Model file for the job. Use its own axes, mm. Coordinates: 2 decimals unless noted, no trailing zeros. Write each loop counter-clockwise with the first axis right and the second up, starting at its lowest first coordinate (ties: lowest second). Pieces come first, ordered by that corner, then holes. Notation, with made-up numbers: (53, 54.25) - (111, 54.25) arc R15 ccw to (111, 69.25) - close; hole circle Ø8 at (-31.5, -8.5). An arc over 180 degrees is marked (long way). Put each result on its own line as item: value. Start each with the question number.
1. Saw through at B-B, the plane y = 137.5. Write the cut outline in (x, z), plus the area to 3 significant figures.
2. Saw through at A-A, the plane z = 9. Write the cut outline in (x, y), plus the area to 3 significant figures.
3. Drop flat-ended pins along their axis: P1, Ø1.5, axis at x = 9.5, y = 92, coming from the +Z side; P2, Ø1, axis at y = 118.5, z = 6, coming from the +X side; P3, Ø4, axis at y = 170.5, z = -11, coming from the -X side. Give the stop position or say it passes through.
4. Saw through at D-D, the plane y = 15. Write the cut outline in (x, z).
5. Saw through at C-C, the plane z = -6.5. Write the cut outline in (x, y).
6. Drill centre lines: L1, parallel to Y at x = 0, z = -4.5; L2, parallel to Y at x = 1, z = 5; L3, parallel to X at y = 15, z = 0. Where is each one in solid material? Low to high. Write a range as from..to.
```python
from build123d import *

# Parameters (mm, degrees)
SKETCH1_W          = 15
SKETCH1_H          = 210
SKETCH3_R          = 3.25
CUT_EXTRUDE1_DEPTH = 212.068709192


with BuildPart() as part:
    # Sketch1 → Revolve1 (revolve)
    with BuildSketch(Plane.XY, mode=Mode.PRIVATE) as revolve1_sk:
        with Locations((-7.5, 105)):
            Rectangle(SKETCH1_W, SKETCH1_H)
    revolve(revolve1_sk.sketch.rotate(Axis((0, 0, 0), (0, 1, 0)), 270), axis=Axis((0, 0, 0), (0, 1, 0)))

    # Sketch3 → Cut-Extrude1 (cut, symmetric)
    with BuildSketch(Plane.XY):
        with Locations((0, 195)):
            Circle(SKETCH3_R)
    cut_extrude1 = extrude(amount=CUT_EXTRUDE1_DEPTH, both=True, mode=Mode.SUBTRACT)

    # Mirror1: Cut-Extrude1 across plane
    add(cut_extrude1.mirror(Plane.ZX.offset(105)), mode=Mode.SUBTRACT)


solid = part.part
```
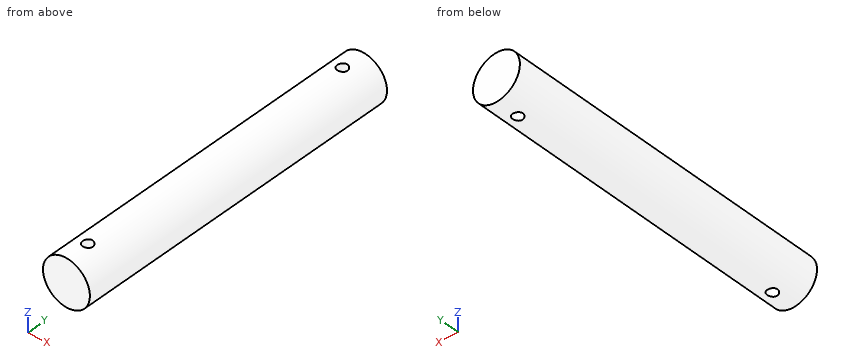
Final values:
1. outline: circle Ø30 at (0, 0)
1. area: 707 mm²
2. outline: (-12, 0) - (12, 0) - (12, 210) - (-12, 210) - close; hole circle Ø6.5 at (0, 15); hole circle Ø6.5 at (0, 195)
2. area: 4,970 mm²
3. P1: stops at z = 12.18
3. P2: stops at x = 13.96
3. P3: stops at x = -12
4. outline: (-3.25, -14.64) - (-3.25, 14.64) arc R15 ccw to start; (3.25, -14.64) arc R15 ccw to (3.25, 14.64) - close
5. outline: (-13.52, 0) - (13.52, 0) - (13.52, 210) - (-13.52, 210) - close; hole circle Ø6.5 at (0, 15); hole circle Ø6.5 at (0, 195)
6. L1: y = 0..11.75, 18.25..191.75, 198.25..210
6. L2: y = 0..11.91, 18.09..191.91, 198.09..210
6. L3: x = -15..-3.25, 3.25..15
